Answer from the drawing. Dimensions are ordinates in mm from the lowest x, y and z of the part. Give positions to 0.01 mm unless a question says otherwise; leave off trailing zeros. Loops run counter-clockwise (first coordinate to the right, second up) from the corner with the lowest first, then second, coordinate; pieces in that order, holes last. Notation, with made-up numbers: (29, -34.5) - (53, -34.5) arc R22 ccw to (53, -9.5) - close; hole circle Ø1 at (71, -29.5). An arc over 180 degrees is marked (long way). Put each result on its own line as item: value. Start each with the question number.
1. Consider L1, parallel to X at y = 43.5, z = 0.6; L2, parallel to X at y = 31, z = 3.2; L3, parallel to Y at x = 105.5, z = 4.4. Determine where each line is inside the solid, lowest interval first. Write a range as from..to.
2. A cutting plane is placed at A-A, the plane z = 3.4. Determine the outline of the cut face in (x, y).
3. A cutting plane is placed at C-C, the plane x = 99. Determine the outline of the cut face in (y, z).
4. Given pin 1 Ø1.5 at (y, z) = (44, 2) entering from +X; pin 2 Ø2.5 at (x, z) = (2.5, 2) entering from +Y; pin 3 Ø2.5 at (y, z) = (44.5, 3.5) entering from -X, each flat-ended and moving along its own axis, determine where each tip first touches the part or whether it passes through.
5. A cutting plane is placed at B-B, the plane y = 63.5. Determine the outline of the cut face in (x, z), plus the area to 4 significant figures.
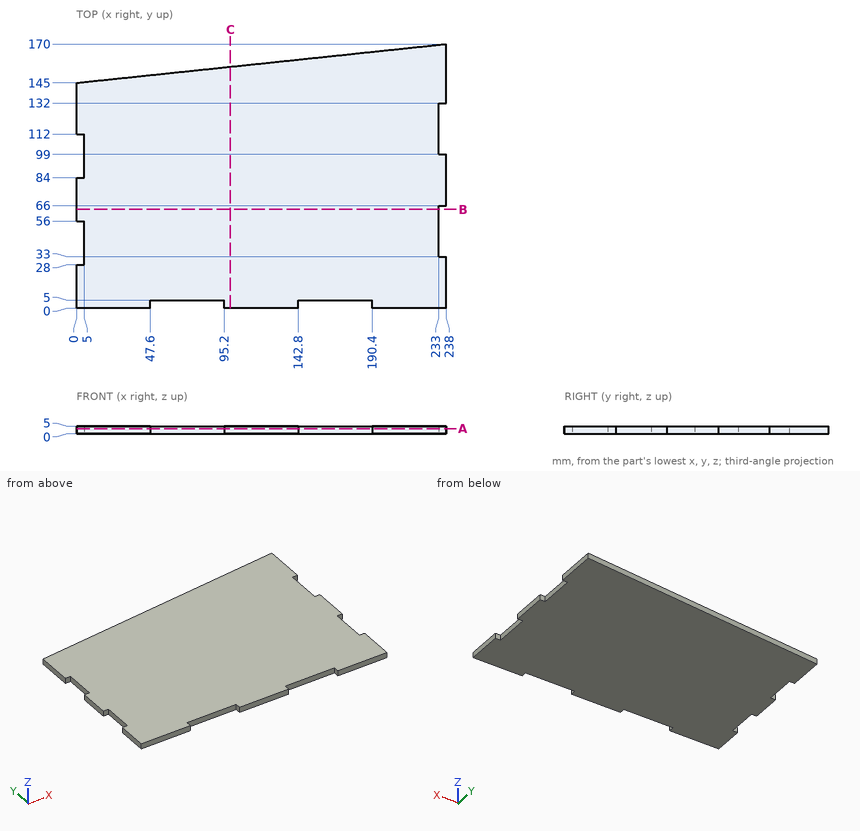
Return value:
1. L1: x = 5..233
1. L2: x = 5..238
1. L3: y = 0..156.08
2. outline: (0, 0) - (47.6, 0) - (47.6, 5) - (95.2, 5) - (95.2, 0) - (142.8, 0) - (142.8, 5) - (190.4, 5) - (190.4, 0) - (238, 0) - (238, 33) - (233, 33) - (233, 66) - (238, 66) - (238, 99) - (233, 99) - (233, 132) - (238, 132) - (238, 170) - (0, 145) - (0, 112) - (5, 112) - (5, 84) - (0, 84) - (0, 56) - (5, 56) - (5, 28) - (0, 28) - close
3. outline: (0, 0) - (155.4, 0) - (155.4, 5) - (0, 5) - close
4. pin 1: stops at x = 233
4. pin 2: stops at y = 145.39
4. pin 3: stops at x = 5
5. outline: (0, 0) - (233, 0) - (233, 5) - (0, 5) - close
5. area: 1,165 mm2
